Part model, mm, in its own coordinate system. Round coordinates to 2 decimals unless told otherwise and drop trailing zeros. Loops run counter-clockwise (first coordinate to the right, second up) from the corner with the lowest first, then second, coordinate; pieces in that order, holes last. Notation, with made-up numbers: (-2, 5.25) -> (12, 5.25) arc R34 cw to (12, 37.25) -> close; hole circle Ø10 at (-1.75, -0.75). An arc over 180 degrees is marked (long way). Answer as a JSON object with one key per item and string values. Group by question number.
from build123d import *

# Parameters (mm, degrees)
SKETCH1_R           = 1.905
BOSS_EXTRUDE1_DEPTH = 50.8
CHAMFER1_SIZE       = 0.508


with BuildPart() as part:
    # Sketch1 → Boss-Extrude1 (new body)
    with BuildSketch(Plane(origin=(0, 0, 0), x_dir=(1, 0, 0), z_dir=(0, 1, 0))):
        Polygon((3.666174209, 0), (1.833087105, 3.175), (-1.833087105, 3.175), (-3.666174209, 0), (-1.833087105, -3.175), (1.833087105, -3.175), align=None)
        Circle(SKETCH1_R, mode=Mode.SUBTRACT)
    extrude(amount=BOSS_EXTRUDE1_DEPTH)

    # Sketch2 → Cut-Revolve1 (revolve, cut)
    with BuildSketch(Plane.XY):
        Polygon((3.666174209, 0), (3.031174209, 0), (3.950242751, 0.919068541), align=None)
        Polygon((3.950242751, 49.880931459), (3.666174209, 50.8), (3.031174209, 50.8), align=None)
    revolve(axis=Axis((0, 49.880931459, 0), (0, -1, 0)), mode=Mode.SUBTRACT)

    # Chamfer1
    chamfer1_edges = [part.edges().sort_by_distance(p)[0] for p in [
        (-1.905, 0, 0),
        (-1.905, 50.8, 0),
    ]]
    chamfer(chamfer1_edges, length=CHAMFER1_SIZE)


solid = part.part
Item 1: Band-saw the part on B-B, the plane x = 0. List the corners of the cut face in (y, z) (3 decimals), plus the area to 3 significant figures.
Item 2: Band-saw the part on A-A, the plane y = 28. List the corners of the cut face in (x, z) (3 decimals).
Item 3: Drop a flat-ended pin along its axis: pin 1 Ø1 at (x, y) = (-3, 40) entering from +Z. Give the stop position or say it passes through.
Item 4: Two-plate mould, pull along Z, no slides. Class faces 1 (the face through (-0.41, 25.05, 1.86)), 2 (the face through (0, 25, 3.175)), 3 (the face through (2.76, 25.05, -1.57)): pulls with the +Z half, pulls with the -Z half, needs draft (parallel to the pull), parting line crosses it, or undercut.
Item 5: Drill centre lines: line 1 (X direction, y = 11.5, z = 0) (3 decimals); line 2 (Z direction, x = -0.5, y = 23) (3 decimals); line 3 (Z direction, x = 0, y = 38.5) (3 decimals). Where is each one in solid material? Low to high.
Entries:
{
 "1": {"outline": "(0, -3.031) -> (0.144, -3.175) -> (50.656, -3.175) -> (50.8, -3.031) -> (50.8, -2.413) -> (50.292, -1.905) -> (0.508, -1.905) -> (0, -2.413) -> close; (0, 2.413) -> (0.508, 1.905) -> (50.292, 1.905) -> (50.8, 2.413) -> (50.8, 3.031) -> (50.656, 3.175) -> (0.144, 3.175) -> (0, 3.031) -> close", "area": "128 mm²"},
 "2": {"outline": "(-3.666, 0) -> (-1.833, -3.175) -> (1.833, -3.175) -> (3.666, 0) -> (1.833, 3.175) -> (-1.833, 3.175) -> close; hole circle Ø3.81 at (0, 0)"},
 "3": {"pin 1": "z = 2.02"},
 "4": {"face 1": "undercut", "face 2": "pulls with the +Z half", "face 3": "pulls with the -Z half"},
 "5": {"line 1": "-3.666 to -1.905, 1.905 to 3.666", "line 2": "-3.175 to -1.838, 1.838 to 3.175", "line 3": "-3.175 to -1.905, 1.905 to 3.175"}
}
